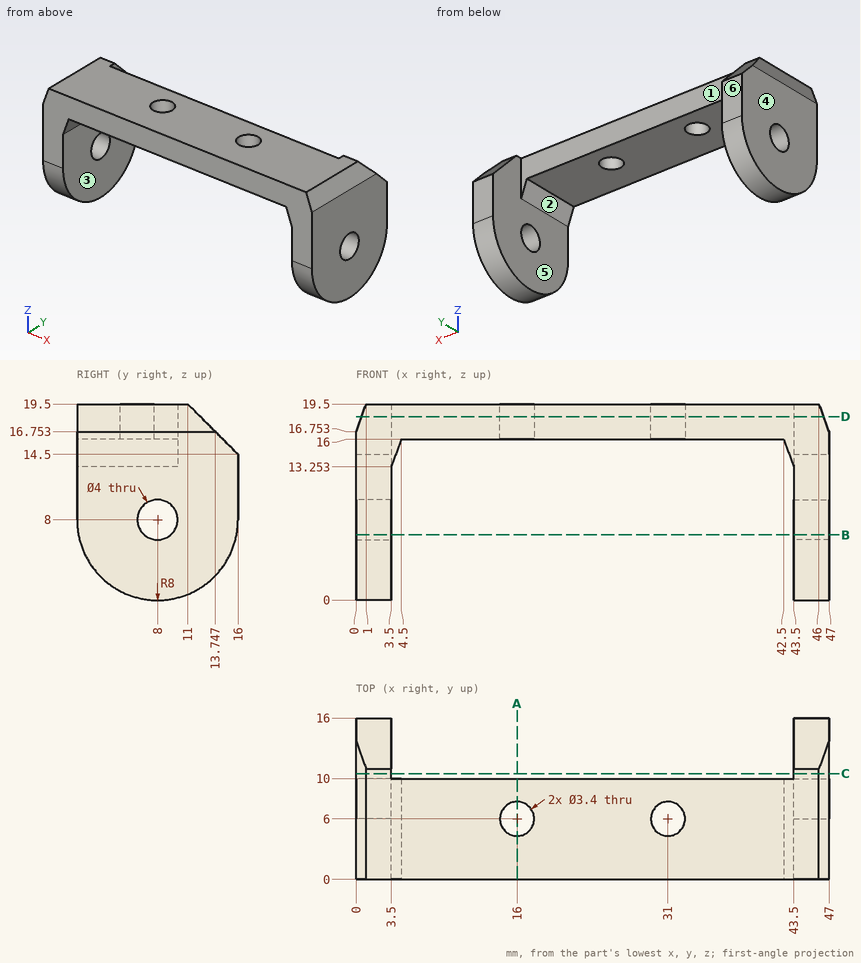
The drawing under review shows one solid part. Ordinate dimensions are in mm from its lowest x, y, z. A direction names the side the tool comes from. Coordinates: 2 decimals unless noted, no trailing zeros. Loops run counter-clockwise (first coordinate to the right, second up) from the corner with the lowest first, then second, coordinate; pieces in that order, holes last. Notation, with made-up numbers: M 30,75.5 L 56,75.5 A25 cw 56,94.5 Z; hole C 78,76.5 d11. An arc over 180 degrees is marked long. Use one line per item in the form item = value.
(1) Consider section D-D (z = 18.25). Give the number of separate pieces and of enclosed holes in the cut face, and give its area (3 significant figures).
Return value:
separate_pieces = 1
enclosed_holes = 2
area = 454 mm2
(2) Consider section C-C (y = 10.5). Write out the cut boundary in (x, z).
Return value:
outline = M 0,0.4 L 3.5,0.4 L 3.5,19.5 L 1,19.5 L 0,16.75 Z; M 43.5,0.4 L 47,0.4 L 47,16.75 L 46,19.5 L 43.5,19.5 Z
(3) For the marked faces 1, 2 and 3, list the 3-axis set-ups (+Z, -Z, +X, -X, +Y, -Y) from which the entire face can be reached by the end or side of a thin tool; tool diameter is ignored.
Return value:
face_1 = +Z, -Z, +Y
face_2 = -Z, +Y, -Y
face_3 = -Z, +Y
(4) Clearance check with flat-ended pins moving along their axes: P1, Ø3, axis at y = 3, z = 8.5, coming from the -X side; P2, Ø5, axis at x = 13.5, z = 15.5, coming from the +Y side; P3, Ø5, axis at x = 26.5, y = 6.5, coming from the -Z side. State where each tip first meets the part, or that it passes through.
Return value:
P1 = 0
P2 = 10
P3 = 16
(5) Draft analysis for pull direction X (two halves, no side actions). For the marked faces 4, 5 and 6, state which applies: pulls with the +X half, pulls with the -X half, needs draft (parallel to the pull), parting line crosses it, or undercut.
Return value:
face_4 = pulls with the -X half
face_5 = undercut
face_6 = needs draft
(6) Consider section A-A (x = 16). Write out the cut boundary in (y, z), and give its area (3 significant figures).
Return value:
outline = M 0,16 L 4.3,16 L 4.3,19.5 L 0,19.5 Z; M 7.7,16 L 10,16 L 10,19.5 L 7.7,19.5 Z
area = 23.1 mm2
(7) For line 1 along X through (y, z) = (6.25, 2); line 2 along Y through (x, z) = (16, 17.75); line 3 along Y through (x, z) = (1.25, 8), list the stretches that pass through material, from the lowest coordinate up. Write a range as from..to.
Return value:
line_1 = 0..3.5, 43.5..47
line_2 = 0..4.3, 7.7..10
line_3 = 0..6, 10..16
(8) Consider section B-B (z = 6.5). Write out the cut boundary in (x, y).
Return value:
outline = M 0,0.14 L 3.5,0.14 L 3.5,6.68 L 0,6.68 Z; M 0,9.32 L 3.5,9.32 L 3.5,15.86 L 0,15.86 Z; M 43.5,0.14 L 47,0.14 L 47,6.68 L 43.5,6.68 Z; M 43.5,9.32 L 47,9.32 L 47,15.86 L 43.5,15.86 Z
